Here's the drawing with two shaded views (mm, measured from the low corner). I have some questions. A direction names the side the tool comes from. Coordinates: 2 decimals unless noted, no trailing zeros. Write each loop counter-clockwise with the first axis right and the second up, starting at its lowest first coordinate (ties: lowest second). Pieces come first, ordered by that corner, then holes. Notation, with made-up numbers: M 86,54 L 130,54 A23 cw 130,69 Z; hole C 70,57 d4. An arc over 180 degrees is marked long. Use one line per item in the form item = value. Start each with the question number.
1. I want a section at A-A, the plane z = 4. List the corners of the cut face in (x, y) for me.
2. I want a section at C-C, the plane y = 25.5. List the corners of the cut face in (x, z) for me (1 decimal).
3. Please list where these lines run through material, in increasing order: line 1 along Y through (x, z) = (18, 3.5); line 2 along Y through (x, z) = (35, 20); line 3 along X through (y, z) = (14.5, 12.5). Write a range as [from, to].
4. I want a section at D-D, the plane x = 10.5. List the corners of the cut face in (y, z) for me, plus the area to 3 significant figures.
5. I want a section at B-B, the plane x = 21. List the corners of the cut face in (y, z) for me (1 decimal).
6. I'm going to push flat-ended pins straight in: pin 1 Ø7.5 at (y, z) = (47, 7.5) entering from +X; pin 2 Ø7.5 at (x, z) = (19.5, 3) entering from -Y; pin 3 Ø14 at (x, y) = (21.5, 22.5) entering from -Z (1 decimal). Where does each tip first touch, or does it pass through?
7. On a 3-axis mill with a long thin cutter (end or side, diameter ignored), from which of +Z, -Z, +X, -X, +Y, -Y can I reach the whole of each face in a straight line? I mean the marked faces 1, 2, 3 and 4. Say none if no direction works.
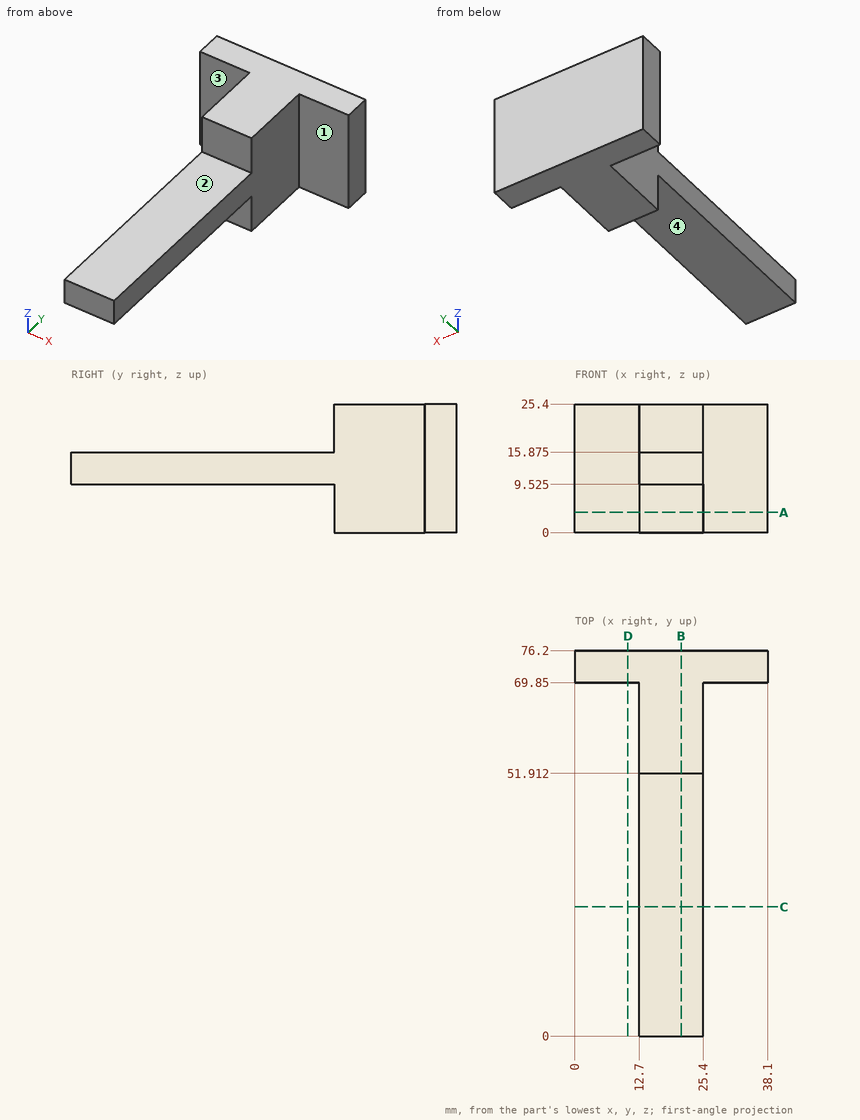
Answer list:
q1.outline = M 0,69.85 L 12.7,69.85 L 12.7,51.91 L 25.4,51.91 L 25.4,69.85 L 38.1,69.85 L 38.1,76.2 L 0,76.2 Z
q2.outline = M 12.7,9.5 L 25.4,9.5 L 25.4,15.9 L 12.7,15.9 Z
q3.line_1 = [51.91, 76.2]
q3.line_2 = [69.85, 76.2]
q3.line_3 = [12.7, 25.4]
q4.outline = M 69.85,0 L 76.2,0 L 76.2,25.4 L 69.85,25.4 Z
q4.area = 161 mm²
q5.outline = M 0,9.5 L 51.9,9.5 L 51.9,0 L 76.2,0 L 76.2,25.4 L 51.9,25.4 L 51.9,15.9 L 0,15.9 Z
q6.pin_1 = 25.4
q6.pin_2 = 51.91
q6.pin_3 = 9.5
q7.face_1 = +Z, -Z, +X, -Y
q7.face_2 = +Z, +X, -X, -Y
q7.face_3 = +Z, -Z, -X, -Y
q7.face_4 = -Z, +X, -X, -Y
